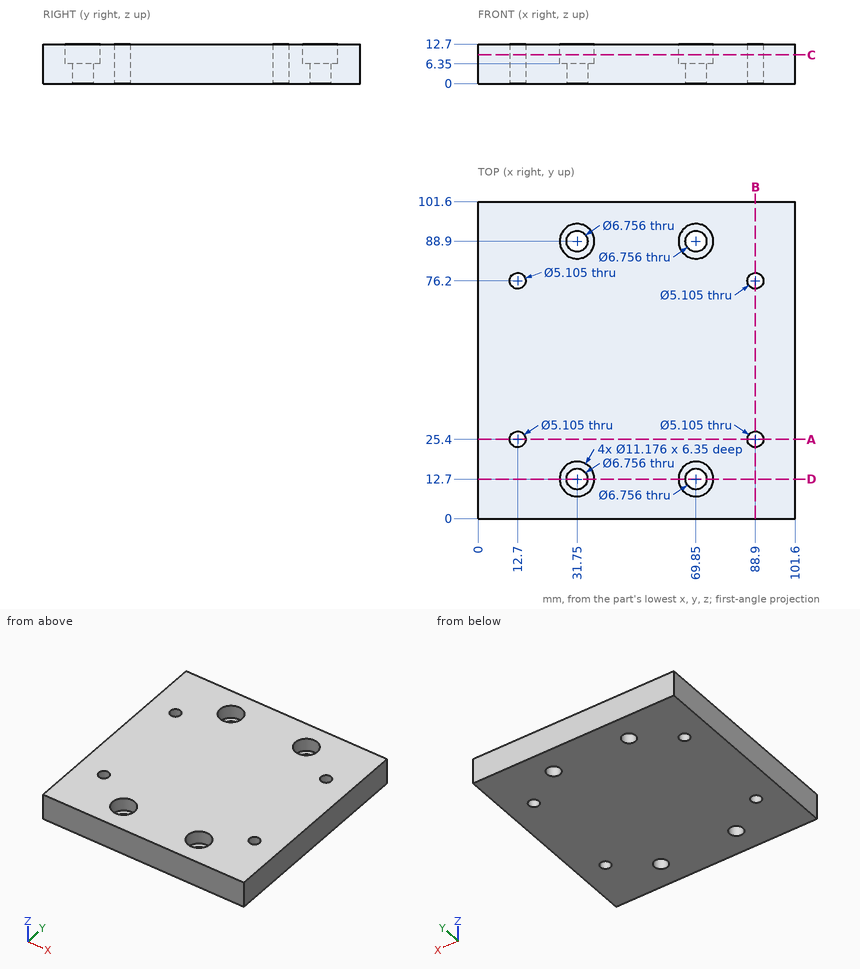
Answer from the drawing. Dimensions are ordinates in mm from the lowest x, y and z of the part. Give positions to 0.01 mm unless a question says otherwise; leave off trailing zeros. Loops run counter-clockwise (first coordinate to the right, second up) from the corner with the lowest first, then second, coordinate; pieces in that order, holes last.
Item 1: Find the intervals of material crossed by line 1 along Y through (x, z) = (12.7, 3.5); line 2 along Y through (x, z) = (31.75, 2); line 3 along Z through (x, y) = (37, 88), in increasing order.
Item 2: The part is cut by section C-C (z = 9.25). Give the number of separate pieces and of enclosed holes in the cut face, and give its area (3 significant figures).
Item 3: The part is cut by section B-B (x = 88.9). Write down the section's boundary in (y, z), and give its area (3 significant figures).
Item 4: Each of these flat-tipped pins is pushed along its axis until it touches: pin 1 Ø4 at (x, y) = (12.7, 76.2) entering from +Z; pin 2 Ø5.5 at (x, y) = (31, 13.5) entering from +Z. Where does it stop, or does it pass through?
Item 5: The part is cut by section A-A (y = 25.4). Write down the section's boundary in (x, z), and give its area (3 significant figures).
Item 6: The part is cut by section D-D (y = 12.7). Write down the section's boundary in (x, z), and give its area (3 significant figures).
Taken from the geometry:
1. line 1: y = 0 to 22.85, 27.95 to 73.65, 78.75 to 101.6
1. line 2: y = 0 to 9.32, 16.08 to 85.52, 92.28 to 101.6
1. line 3: z = 0 to 6.35
2. separate pieces: 1
2. enclosed holes: 8
2. area: 9,850 mm2
3. outline: (0, 0) - (22.85, 0) - (22.85, 12.7) - (0, 12.7) - close; (27.95, 0) - (73.65, 0) - (73.65, 12.7) - (27.95, 12.7) - close; (78.75, 0) - (101.6, 0) - (101.6, 12.7) - (78.75, 12.7) - close
3. area: 1,160 mm2
4. pin 1: passes through
4. pin 2: stops at z = 6.35
5. outline: (0, 0) - (10.15, 0) - (10.15, 12.7) - (0, 12.7) - close; (15.25, 0) - (86.35, 0) - (86.35, 12.7) - (15.25, 12.7) - close; (91.45, 0) - (101.6, 0) - (101.6, 12.7) - (91.45, 12.7) - close
5. area: 1,160 mm2
6. outline: (0, 0) - (28.37, 0) - (28.37, 6.35) - (26.16, 6.35) - (26.16, 12.7) - (0, 12.7) - close; (35.13, 0) - (66.47, 0) - (66.47, 6.35) - (64.26, 6.35) - (64.26, 12.7) - (37.34, 12.7) - (37.34, 6.35) - (35.13, 6.35) - close; (73.23, 0) - (101.6, 0) - (101.6, 12.7) - (75.44, 12.7) - (75.44, 6.35) - (73.23, 6.35) - close
6. area: 1,060 mm2
